Build history of the part. All positions in model axes, mm. A direction names the side the tool comes from. Give positions to 0.01 mm unless a question says otherwise; leave off trailing zeros. Order: outer loops, then holes, each group sorted by start corner. A loop starts at its lowest first (then second) coordinate and runs counter-clockwise, first axis right, second up. Notation, with made-up numbers: (50.25, 83) -> (66.25, 83) arc R16 cw to (66.25, 108) -> close; hole circle Ø4 at (-22.5, 18). An arc over 180 degrees is marked (long way). One line per item, written item: value. Start each with the question number.
(1) Two-plate mould, pull along X, no slides. Class faces 4 (the cylindrical face through (18.52, 9.82, -28.61)), 5 (the flat face through (58, 6, -29)), 6 (the flat face through (55, 6, -29)): +X half, -X half, draft (parallel to the pull), parting line (faces both ways), or undercut.
(2) Probe line 1 (Y direction, x = 18.4, z = -31); line 2 (X direction, y = 1.05, z = -26.5); line 3 (Y direction, x = 41.5, z = -2). List the from-to ranges inside material, lowest first.
(3) Which spindle directions (+Z, -Z, +X, -X, +Y, -Y) get a long thin tool onto all of the face, cutting with end or side? Do faces 1 (the flat face through (57, 3.01, -31)), 2 (the flat face through (17, 6, -29)), 3 (the flat face through (20, 6, -29)). Say none if no direction does.
(4) Saw through at B-B on x = 62.5. Give the cut face in (y, z).
(5) Pin check, flat tips, straight feed: pin 1 (0.7 mm diameter, centred on x = 56.5, z = -31, fed in from -Y); pin 2 (2.5 mm diameter, centred on y = 7, z = -27, fed in from +X); pin 3 (1.5 mm diameter, centred on x = 52, z = -27.5, fed in from +Y). Stop position of each tip, or through.
(6) Saw through at C-C on x = 36.5. Give the cut face in (y, z).
(7) Saw through at A-A on z = -31. Give the cut face in (x, y).
(8) Saw through at D-D on x = 52. Give the cut face in (y, z), plus the area to 3 significant figures.
```python
from build123d import *

# Parameters (mm, degrees)
SKETCH1_W            = 75
SKETCH1_H            = 30
BOSS_EXTRUDE1_DEPTH  = 2
M3_CLEARANCE_HOLE1_D = 3.6
SKETCH4_R            = 1.75
BOSS_EXTRUDE2_DEPTH  = 3
BOSS_EXTRUDE3_START  = -38
SKETCH4_2_R          = 1.75
BOSS_EXTRUDE3_DEPTH  = 3
FILLET1_R            = 2
M3_CLEARANCE_HOLE2_D = 3.6
M3_CLEARANCE_HOLE3_D = 3.6


with BuildPart() as part:
    # Sketch1 → Boss-Extrude1 (new body)
    with BuildSketch(Plane(origin=(0, 0, 0), x_dir=(1, 0, 0), z_dir=(0, 1, 0))):
        with Locations((37.5, 15)):
            Rectangle(SKETCH1_W, SKETCH1_H)
    extrude(amount=BOSS_EXTRUDE1_DEPTH)

    # M3 Clearance Hole1 (through all)
    with Locations(Plane(origin=(0, 2, 0), x_dir=(1, 0, 0), z_dir=(0, 1, 0))):
        with Locations((42.5, 3.7), (32.5, 3.7), (22.5, 3.7), (12.5, 3.7), (62.5, 3.7), (52.5, 3.7)):
            Hole(M3_CLEARANCE_HOLE1_D / 2)

    # Sketch4 → Boss-Extrude2 (add)
    # profile 1 of 2: a face of its own
    with BuildSketch(Plane.ZY.offset(-20)):
        with BuildLine():
            ThreePointArc((-29.462001252, 10.010018789), (-28.595073643, 9.812360744), (-27.899501252, 9.258455311))
            Line((-27.899501252, 9.258455311), (-22.1, 2))
            Line((-22.1, 2), (-28.5, 2))
            Line((-28.5, 2), (-28.706505632, 2.258455311))
            ThreePointArc((-28.706505632, 2.258455311), (-29.402078024, 2.812360744), (-30.269005632, 3.010018789))
            Line((-30.269005632, 3.010018789), (-32.55, 3.010018789))
            ThreePointArc((-32.55, 3.010018789), (-33.964213562, 3.595805227), (-34.55, 5.010018789))
            Line((-34.55, 5.010018789), (-34.55, 8.010018789))
            ThreePointArc((-34.55, 8.010018789), (-33.964213562, 9.424232352), (-32.55, 10.010018789))
            Line((-32.55, 10.010018789), (-29.462001252, 10.010018789))
        make_face()
        with Locations((-31, 6.510018789)):
            Circle(SKETCH4_R, mode=Mode.SUBTRACT)
    # profile 2 of 2: a face of its own
    with BuildSketch(Plane.ZY.offset(-20)):
        with Locations((-31, 6.510018789)):
            Circle(SKETCH4_R)
    extrude(amount=BOSS_EXTRUDE2_DEPTH)

    # Sketch4<2> → Boss-Extrude3 (add)
    # profile 1 of 2: a face of its own
    with BuildSketch(Plane.ZY.offset(-20).offset(BOSS_EXTRUDE3_START)):
        with BuildLine():
            ThreePointArc((-29.462001252, 10.010018789), (-28.595073643, 9.812360744), (-27.899501252, 9.258455311))
            Line((-27.899501252, 9.258455311), (-22.1, 2))
            Line((-22.1, 2), (-28.5, 2))
            Line((-28.5, 2), (-28.706505632, 2.258455311))
            ThreePointArc((-28.706505632, 2.258455311), (-29.402078024, 2.812360744), (-30.269005632, 3.010018789))
            Line((-30.269005632, 3.010018789), (-32.55, 3.010018789))
            ThreePointArc((-32.55, 3.010018789), (-33.964213562, 3.595805227), (-34.55, 5.010018789))
            Line((-34.55, 5.010018789), (-34.55, 8.010018789))
            ThreePointArc((-34.55, 8.010018789), (-33.964213562, 9.424232352), (-32.55, 10.010018789))
            Line((-32.55, 10.010018789), (-29.462001252, 10.010018789))
        make_face()
        with Locations((-31, 6.510018789)):
            Circle(SKETCH4_2_R, mode=Mode.SUBTRACT)
    # profile 2 of 2: a face of its own
    with BuildSketch(Plane.ZY.offset(-20).offset(BOSS_EXTRUDE3_START)):
        with Locations((-31, 6.510018789)):
            Circle(SKETCH4_2_R)
    extrude(amount=BOSS_EXTRUDE3_DEPTH)

    # Fillet1
    fillet1_edges = [part.edges().sort_by_distance(p)[0] for p in [
        (18.5, 2, -22.1),
        (56.5, 2, -22.1),
    ]]
    fillet(fillet1_edges, radius=FILLET1_R)

    # M3 Clearance Hole2 (through all)
    with Locations(Plane(origin=(58, 0, 0), x_dir=(0, 0, -1), z_dir=(1, 0, 0))):
        with Locations((31, 6.510018789)):
            Hole(M3_CLEARANCE_HOLE2_D / 2)

    # M3 Clearance Hole3 (through all)
    with Locations(Plane(origin=(0, 0, 0), x_dir=(-1, 0, 0), z_dir=(0, -1, 0))):
        with Locations((-49.3, 16.2), (-71.5, 26.5)):
            Hole(M3_CLEARANCE_HOLE3_D / 2)


solid = part.part
```
Results below:
1. face 4: draft
1. face 5: +X half
1. face 6: undercut
2. line 1: y = 3.01 to 4.71, 8.31 to 10.01
2. line 2: x = 0 to 69.7, 73.3 to 75
2. line 3: y = 0 to 2
3. face 1: -Z, +X, -X, -Y
3. face 2: +Z, -Z, -X, +Y
3. face 3: +Z, -Z, +Y
4. outline: (0, -30) -> (2, -30) -> (2, -5.5) -> (0, -5.5) -> close; (0, -1.9) -> (2, -1.9) -> (2, 0) -> (0, 0) -> close
5. pin 1: stops at y = 3.01
5. pin 2: stops at x = 58
5. pin 3: stops at y = 2
6. outline: (0, -30) -> (2, -30) -> (2, 0) -> (0, 0) -> close
7. outline: (17, 3.01) -> (20, 3.01) -> (20, 4.71) -> (17, 4.71) -> close; (17, 8.31) -> (20, 8.31) -> (20, 10.01) -> (17, 10.01) -> close; (55, 3.01) -> (58, 3.01) -> (58, 4.71) -> (55, 4.71) -> close; (55, 8.31) -> (58, 8.31) -> (58, 10.01) -> (55, 10.01) -> close
8. outline: (0, -30) -> (2, -30) -> (2, -5.43) -> (0, -5.43) -> close; (0, -1.97) -> (2, -1.97) -> (2, 0) -> (0, 0) -> close
8. area: 53.1 mm²
